Geometry: final body of the model. Coordinates: model frame, mm. Face numbers are marked on the shaded views. A direction names the side the tool comes from. Give positions to 0.01 mm unless a question says otherwise; leave off trailing zeros. Order: outer loops, then holes, each group sorted by start corner. A loop starts at its lowest first (then second) coordinate and runs counter-clockwise, first axis right, second up. Notation, with made-up numbers: (12, -37.75) -> (31, -37.75) arc R22 cw to (31, -21.75) -> close; hole circle Ø11 at (72.5, 16.25). An arc over 180 degrees is marked (long way). One line per question, with ' | ' between items. Start each with the question number.
(1) First-contact query: pin 1 Ø1.4 at (y, z) = (101, 55.5) entering from -X; pin 2 Ø0.8 at (y, z) = (94, 53.5) entering from +X; pin 3 Ø1 at (y, z) = (111.5, 56) entering from +X; pin 4 Ø1.5 at (x, y) = (-13, 103) entering from +Z. Flat tips, straight axial feed; report the tip coordinate or a pass-through.
(2) Section A-A (y = 113). Return loops of the section in (x, z).
(3) Set-up query: the marked faces 1 and 2. Return all of +Z, -Z, +X, -X, +Y, -Y with unobstructed straight access to the full face (end or side cutting, diameter ignored); none if empty.
(4) Section B-B (z = 53.25). State how many separate pieces and enclosed holes the cut face has, then the cut area to 3 significant figures.
(5) Ray query, L1, parallel to Y at x = -3.5, z = 55.75; L2, parallel to Y at x = -47, z = 56; L3, parallel to Y at x = -20, z = 53.75. Return the intervals inside material, ascending.
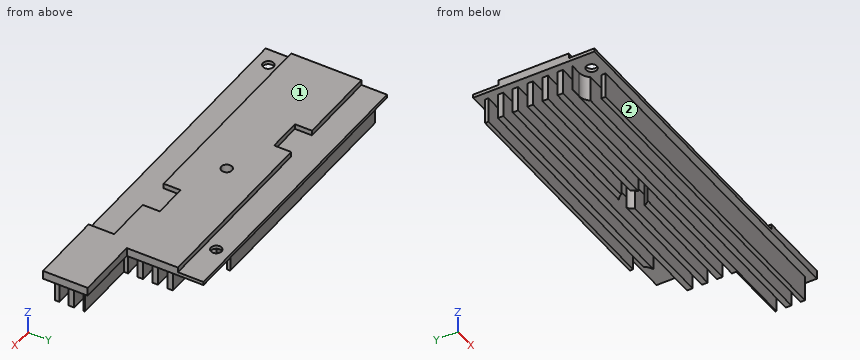
```python
from build123d import *

# Parameters (mm, degrees)
BOSS_EXTRU_1_DEPTH      = 2
BOSS_EXTRU_2_DEPTH      = 6
ESQUISSE3_R             = 1.25
ENL_V_MAT_EXTRU_1_DEPTH = 148.965253472
ESQUISSE4_R             = 2.915475947
ENL_V_MAT_EXTRU_2_DEPTH = 6
ENL_V_MAT_EXTRU_3_DEPTH = 1.2
ESQUISSE12_W            = 85.5
ESQUISSE12_H            = 2.2
ENL_V_MAT_EXTRU_4_DEPTH = 6


with BuildPart() as part:
    # Esquisse1 → Boss.-Extru.1 (new body)
    with BuildSketch(Plane(origin=(0, 0, 59.701801036), x_dir=(-1, 0, 0), z_dir=(0, 0, -1))):
        Polygon((0.68526114, 91.507570583), (86.18526114, 91.507570583), (86.18526114, 120.007570583), (15.68526114, 120.007570583), (15.68526114, 102.007570583), (0.68526114, 102.007570583), align=None)
    extrude(amount=BOSS_EXTRU_1_DEPTH)

    # Esquisse2 → Boss.-Extru.2 (add)
    with BuildSketch(Plane(origin=(0, 0, 57.701801036), x_dir=(-1, 0, 0), z_dir=(0, 0, -1))):
        Polygon((84.43526114, 93.257570583), (84.43526114, 118.257570583), (17.43526114, 118.257570583), (17.43526114, 100.257570583), (2.43526114, 100.257570583), (2.43526114, 93.257570583), align=None)
    extrude(amount=BOSS_EXTRU_2_DEPTH)

    # Esquisse3 → Enlèv. mat.-Extru.1 (cut, through all)
    with BuildSketch(Plane(origin=(0, 0, 51.701801036), x_dir=(-1, 0, 0), z_dir=(0, 0, -1))):
        with Locations((47.93526114, 105.757570583)):
            Circle(ESQUISSE3_R)
        with Locations((25.93526114, 116.757570583)):
            Circle(ESQUISSE3_R)
        with Locations((81.93526114, 94.757570583)):
            Circle(ESQUISSE3_R)
    extrude(amount=-ENL_V_MAT_EXTRU_1_DEPTH, mode=Mode.SUBTRACT)

    # Esquisse4 → Enlèv. mat.-Extru.2 (cut)
    with BuildSketch(Plane(origin=(0, 0, 51.701801036), x_dir=(-1, 0, 0), z_dir=(0, 0, -1))):
        with Locations((47.93526114, 105.757570583)):
            Circle(ESQUISSE4_R)
        with BuildLine():
            Line((25.93526114, 113.842094636), (17.43526114, 113.842094636))
            Line((17.43526114, 113.842094636), (17.43526114, 118.257570583))
            Line((17.43526114, 118.257570583), (28.850737087, 118.257570583))
            Line((28.850737087, 118.257570583), (28.850737087, 116.757570583))
            ThreePointArc((28.850737087, 116.757570583), (27.996813953, 114.696017771), (25.93526114, 113.842094636))
        make_face()
        with BuildLine():
            Line((79.019785192, 94.757570583), (79.019785192, 91.842094636))
            Line((79.019785192, 91.842094636), (84.850737087, 91.842094636))
            Line((84.850737087, 91.842094636), (84.850737087, 97.673046531))
            Line((84.850737087, 97.673046531), (81.93526114, 97.673046531))
            ThreePointArc((81.93526114, 97.673046531), (79.873708327, 96.819123396), (79.019785192, 94.757570583))
        make_face()
    extrude(amount=-ENL_V_MAT_EXTRU_2_DEPTH, mode=Mode.SUBTRACT)

    # Esquisse11 → Enlèv. mat.-Extru.3 (cut)
    with BuildSketch(Plane.XY.offset(59.701801036)):
        Polygon((-18.18526114, 91.507570583), (-18.18526114, 97.507570583), (-29.18526114, 97.507570583), (-29.18526114, 101.507570583), (-37.18526114, 101.507570583), (-37.18526114, 97.507570583), (-86.18526114, 97.507570583), (-86.18526114, 91.507570583), align=None)
        Polygon((-15.68526114, 114.007570583), (-59.18526114, 114.007570583), (-59.18526114, 110.007570583), (-67.18526114, 110.007570583), (-67.18526114, 114.007570583), (-86.18526114, 114.007570583), (-86.18526114, 120.007570583), (-15.68526114, 120.007570583), align=None)
    extrude(amount=-ENL_V_MAT_EXTRU_3_DEPTH, mode=Mode.SUBTRACT)

    # Esquisse12 → Enlèv. mat.-Extru.4 (cut)
    with BuildSketch(Plane(origin=(0, 0, 51.701801036), x_dir=(-1, 0, 0), z_dir=(0, 0, -1))):
        with Locations((43.43526114, 95.357570583)):
            Rectangle(ESQUISSE12_W, ESQUISSE12_H)
        with Locations((43.43526114, 98.857570583)):
            Rectangle(ESQUISSE12_W, ESQUISSE12_H)
        with Locations((43.43526114, 102.357570583)):
            Rectangle(ESQUISSE12_W, ESQUISSE12_H)
        with Locations((43.43526114, 105.857570583)):
            Rectangle(ESQUISSE12_W, ESQUISSE12_H)
        with Locations((43.43526114, 109.357570583)):
            Rectangle(ESQUISSE12_W, ESQUISSE12_H)
        with Locations((43.43526114, 112.857570583)):
            Rectangle(ESQUISSE12_W, ESQUISSE12_H)
        with Locations((43.43526114, 116.357570583)):
            Rectangle(ESQUISSE12_W, ESQUISSE12_H)
    extrude(amount=-ENL_V_MAT_EXTRU_4_DEPTH, mode=Mode.SUBTRACT)


solid = part.part
```
Response:
1) pin 1: stops at x = -84.44 | pin 2: stops at x = -2.44 | pin 3: stops at x = -17.44 | pin 4: passes through
2) outline: (-86.19, 57.7) -> (-15.69, 57.7) -> (-15.69, 59.7) -> (-59.19, 59.7) -> (-59.19, 58.5) -> (-67.19, 58.5) -> (-67.19, 59.7) -> (-86.19, 59.7) -> close
3) face 1: +Z, +X, -X, +Y, -Y | face 2: -Z, +X, -X, -Y
4) separate pieces: 10 | enclosed holes: 0 | area: 637 mm^2
5) L1: y = 93.26 to 94.26, 96.46 to 97.76, 99.96 to 100.26 | L2: y = 93.26 to 94.26, 96.46 to 97.76, 99.96 to 101.26, 110.46 to 111.76, 113.96 to 115.26, 117.46 to 118.26 | L3: y = 93.26 to 94.26, 96.46 to 97.76, 99.96 to 101.26, 103.46 to 104.76, 106.96 to 108.26, 110.46 to 111.76
